Print and shaded views of the part. All mm, measured from the part's lowest x, y and z. Give positions to 0.01 mm unless a question says otherwise; leave off trailing zeros. Write each loop counter-clockwise with the first axis right and the second up, starting at its lowest first coordinate (ties: lowest second). Pieces come first, ordered by that corner, then holes.
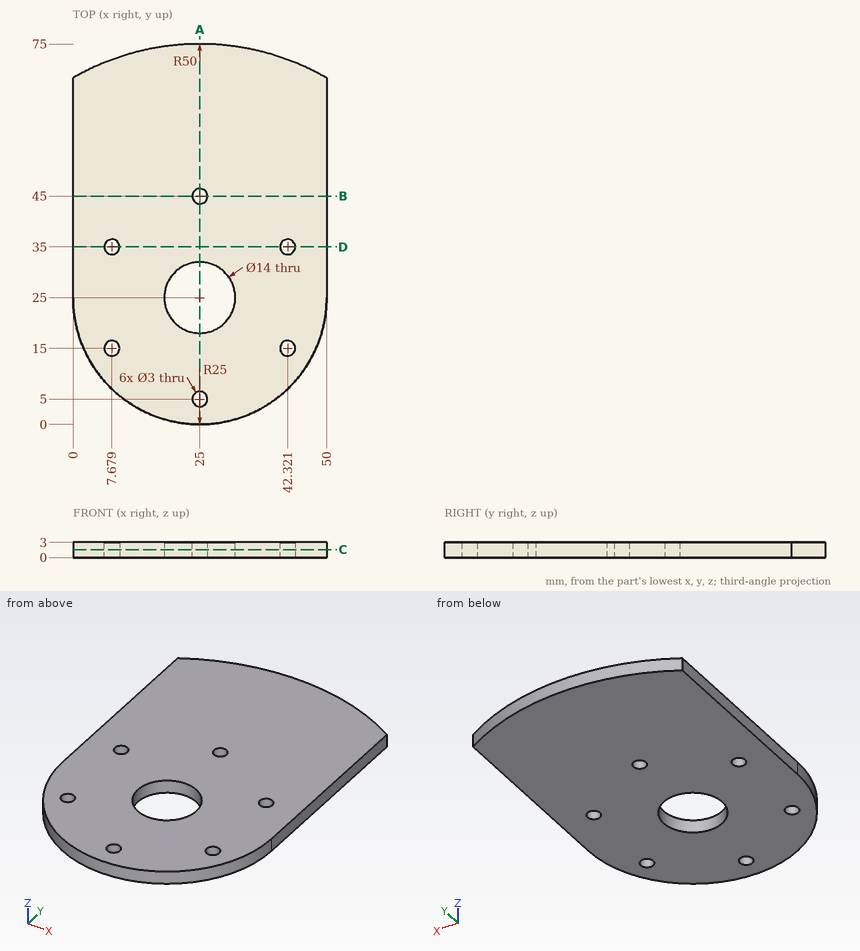
1. Saw through at A-A on x = 25. Give the cut face in (y, z), plus the area to 3 significant figures.
2. Drop a flat-ended pin along its axis: pin 1 (1 mm diameter, centred on x = 35.5, z = 1.5, fed in from -Y). Give the stop position or say it passes through.
3. Saw through at D-D on y = 35. Give the cut face in (x, z), plus the area to 3 significant figures.
4. Saw through at C-C on z = 1.6. Give the cut face in (x, y).
5. Drill centre lines: line 1 along Y through (x, z) = (25, 0.85); line 2 along Y through (x, z) = (42, 1) (1 decimal); line 3 along X through (y, z) = (22, 1.5) (1 decimal). Where is each one in solid material? Low to high.
6. Saw through at B-B on y = 45. Give the cut face in (x, z), plus the area to 3 significant figures.
Outcome:
1. outline: (0, 0) - (3.5, 0) - (3.5, 3) - (0, 3) - close; (6.5, 0) - (18, 0) - (18, 3) - (6.5, 3) - close; (32, 0) - (43.5, 0) - (43.5, 3) - (32, 3) - close; (46.5, 0) - (75, 0) - (75, 3) - (46.5, 3) - close
1. area: 165 mm2
2. pin 1: stops at y = 2.09
3. outline: (0, 0) - (6.18, 0) - (6.18, 3) - (0, 3) - close; (9.18, 0) - (40.82, 0) - (40.82, 3) - (9.18, 3) - close; (43.82, 0) - (50, 0) - (50, 3) - (43.82, 3) - close
3. area: 132 mm2
4. outline: (0, 25) arc R25 ccw to (50, 25) - (50, 68.3) arc R50 ccw to (0, 68.3) - close; hole circle Ø3 at (7.68, 15); hole circle Ø3 at (7.68, 35); hole circle Ø14 at (25, 25); hole circle Ø3 at (25, 5); hole circle Ø3 at (25, 45); hole circle Ø3 at (42.32, 15); hole circle Ø3 at (42.32, 35)
5. line 1: y = 0 to 3.5, 6.5 to 18, 32 to 43.5, 46.5 to 75
5. line 2: y = 6.7 to 13.5, 16.5 to 33.5, 36.5 to 72
5. line 3: x = 0.2 to 18.7, 31.3 to 49.8
6. outline: (0, 0) - (23.5, 0) - (23.5, 3) - (0, 3) - close; (26.5, 0) - (50, 0) - (50, 3) - (26.5, 3) - close
6. area: 141 mm2
